```python
from build123d import *

# Parameters (mm, degrees)
SKETCH_1_R          = 1.5
EXTRUDE_1_DEPTH     = 3
EXTRUDE_2_DEPTH     = 3
SKETCH_3_R          = 1.25
CUT_EXTRUDE_1_DEPTH = 3
SKETCH_4_R          = 0.75
CUT_EXTRUDE_2_DEPTH = 10
CUT_EXTRUDE_START   = -3
SKETCH_5_R          = 2
CUT_EXTRUDE_3_DEPTH = 1


with BuildPart() as part:
    # 草图1 → 凸台-拉伸1 (new body)
    with BuildSketch(Plane.XY):
        with BuildLine():
            Line((-23, 25), (23, 25))
            ThreePointArc((23, 25), (24.414213562, 24.414213562), (25, 23))
            Line((25, 23), (25, -23))
            ThreePointArc((25, -23), (24.414213562, -24.414213562), (23, -25))
            Line((23, -25), (-23, -25))
            ThreePointArc((-23, -25), (-24.414213562, -24.414213562), (-25, -23))
            Line((-25, -23), (-25, 23))
            ThreePointArc((-25, 23), (-24.414213562, 24.414213562), (-23, 25))
        make_face()
        with Locations((-22, 22)):
            Circle(SKETCH_1_R, mode=Mode.SUBTRACT)
        with Locations((22, 22)):
            Circle(SKETCH_1_R, mode=Mode.SUBTRACT)
        with Locations((22, -22)):
            Circle(SKETCH_1_R, mode=Mode.SUBTRACT)
        with Locations((-22, -22)):
            Circle(SKETCH_1_R, mode=Mode.SUBTRACT)
    extrude(amount=EXTRUDE_1_DEPTH)

    # 草图2 → 凸台-拉伸2 (add)
    with BuildSketch(Plane.XY.offset(3)):
        with BuildLine():
            ThreePointArc((2.65, -6.12291072), (6.950358309, -3.476304453), (9.287087811, 1))
            Line((9.287087811, 1), (7.228416147, 1))
            ThreePointArc((7.228416147, 1), (5.53953249, -2.056043887), (2.65, -4.016231182))
            Line((2.65, -4.016231182), (2.65, -6.12291072))
        make_face()
        with BuildLine():
            Line((-7.228416147, 1), (-9.287087811, 1))
            ThreePointArc((-9.287087811, 1), (-6.950358309, -3.476304453), (-2.65, -6.12291072))
            Line((-2.65, -6.12291072), (-2.65, -4.016231182))
            ThreePointArc((-2.65, -4.016231182), (-5.53953249, -2.056043887), (-7.228416147, 1))
        make_face()
        with BuildLine():
            Line((-2.65, 10.016231182), (-2.65, 12.12291072))
            ThreePointArc((-2.65, 12.12291072), (-6.950358309, 9.476304453), (-9.287087811, 5))
            Line((-9.287087811, 5), (-7.228416147, 5))
            ThreePointArc((-7.228416147, 5), (-5.53953249, 8.056043887), (-2.65, 10.016231182))
        make_face()
        with BuildLine():
            ThreePointArc((9.287087811, 5), (6.950358309, 9.476304453), (2.65, 12.12291072))
            Line((2.65, 12.12291072), (2.65, 10.016231182))
            ThreePointArc((2.65, 10.016231182), (5.53953249, 8.056043887), (7.228416147, 5))
            Line((7.228416147, 5), (9.287087811, 5))
        make_face()
    extrude(amount=EXTRUDE_2_DEPTH)

    # 草图3 → 切除-拉伸1 (cut)
    with BuildSketch(Plane.XY.offset(3)):
        with Locations((0, 3)):
            Circle(SKETCH_3_R)
    extrude(amount=-CUT_EXTRUDE_1_DEPTH, mode=Mode.SUBTRACT)

    # 草图4 → 切除-拉伸2 (cut)
    with BuildSketch(Plane.XY.offset(3)):
        with Locations((0, 17.5)):
            Circle(SKETCH_4_R)
        with Locations((0, -11.5)):
            Circle(SKETCH_4_R)
        with Locations((-6.25, 3)):
            Circle(SKETCH_4_R)
        with Locations((6.25, 3)):
            Circle(SKETCH_4_R)
    extrude(amount=-CUT_EXTRUDE_2_DEPTH, mode=Mode.SUBTRACT)

    # 草图5 → 切除-拉伸3 (cut)
    with BuildSketch(Plane(origin=(0, 0, 0), x_dir=(-1, 0, 0), z_dir=(0, 0, -1)).offset(CUT_EXTRUDE_START)):
        with Locations((0, 3)):
            Circle(SKETCH_5_R)
    extrude(amount=CUT_EXTRUDE_3_DEPTH, mode=Mode.SUBTRACT)


solid = part.part
```
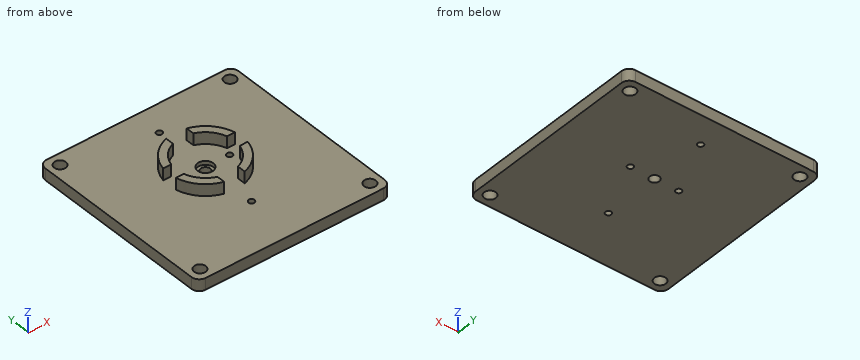
CAD build for the part. Positions are in the model's coordinates, mm. Round coordinates to 2 decimals unless told otherwise and drop trailing zeros. Order: outer loops, then holes, each group sorted by start corner. A loop starts at its lowest first (then second) coordinate and runs counter-clockwise, first axis right, second up.
Item 1: Saw through at D-D on x = 6.25. Write the cut outline in (y, z), then the cut area to 3 significant figures.
Item 2: Saw through at A-A on z = 5.15. Write the cut outline in (x, y), then the cut area to 3 significant figures.
Item 3: Probe line 1 along Y through (x, z) = (0, 1); line 2 along Y through (x, z) = (22, 1.85); line 3 along Y through (x, z) = (6.25, 0.95). List the from-to ranges inside material, lowest first.
Item 4: Pin check, flat tips, straight feed: pin 1 (2 mm diameter, centred on x = -15.5, y = -8.5, fed in from +Z); pin 2 (8 mm diameter, centred on x = -3.5, y = 9.5, fed in from +Z); pin 3 (1.7 mm diameter, centred on y = 11, z = 5, fed in from -X); pin 4 (1.6 mm diameter, centred on x = -8, z = 5, fed in from +Y). Stop position of each tip, or through.
Item 5: Saw through at C-C on y = -11.5. Write the cut outline in (x, z), then the cut area to 4 significant figures.
Item 6: Saw through at B-B on x = -22. Write the cut outline in (y, z).
Reported:
1. outline: (-25, 0) - (2.25, 0) - (2.25, 3) - (-1.15, 3) - (-1.15, 6) - (-4.15, 6) - (-4.15, 3) - (-25, 3) - close; (3.75, 0) - (25, 0) - (25, 3) - (10.15, 3) - (10.15, 6) - (7.15, 6) - (7.15, 3) - (3.75, 3) - close
1. area: 164 mm2
2. outline: (-9.29, 1) arc R9.5 ccw to (-2.65, -6.12) - (-2.65, -4.02) arc R7.5 cw to (-7.23, 1) - close; (-9.29, 5) - (-7.23, 5) arc R7.5 cw to (-2.65, 10.02) - (-2.65, 12.12) arc R9.5 ccw to start; (2.65, -6.12) arc R9.5 ccw to (9.29, 1) - (7.23, 1) arc R7.5 cw to (2.65, -4.02) - close; (2.65, 10.02) arc R7.5 cw to (7.23, 5) - (9.29, 5) arc R9.5 ccw to (2.65, 12.12) - close
2. area: 69.1 mm2
3. line 1: y = -25 to -12.25, -10.75 to 1.75, 4.25 to 16.75, 18.25 to 25
3. line 2: y = -25 to -23.5, -20.5 to 20.5, 23.5 to 25
3. line 3: y = -25 to 2.25, 3.75 to 25
4. pin 1: stops at z = 3
4. pin 2: stops at z = 6
4. pin 3: stops at x = -6.26
4. pin 4: stops at y = 9.2
5. outline: (-25, 0) - (-0.75, 0) - (-0.75, 3) - (-25, 3) - close; (0.75, 0) - (25, 0) - (25, 3) - (0.75, 3) - close
5. area: 145.5 mm2
6. outline: (-25, 0) - (-23.5, 0) - (-23.5, 3) - (-25, 3) - close; (-20.5, 0) - (20.5, 0) - (20.5, 3) - (-20.5, 3) - close; (23.5, 0) - (25, 0) - (25, 3) - (23.5, 3) - close
